Input: part model. Units: mm. Frame: model coordinates. Face numbers are marked on the shaded views. Round coordinates to 2 decimals unless told otherwise and drop trailing zeros. Loops run counter-clockwise (first coordinate to the right, second up) from the corner with the lowest first, then second, coordinate; pieces in that order, holes last. Notation, with made-up numbers: (36.5, 73.25) - (54.5, 73.25) arc R10 cw to (54.5, 89.25) - close; hole circle Ø2 at (69, 3.5). An arc over 180 degrees is marked (long way). One line per question, with ' | ' between items. Start each with the question number.
Item 1: Material intervals for line 1 along Z through (x, y) = (-4.5, 7); line 2 along Y through (x, z) = (-7, -12); line 3 along X through (y, z) = (0, -1), sorted ascending.
Item 2: Section C-C, the plane x = 3. Return loops of the section in (y, z).
Item 3: Section D-D, the plane z = -5. Return loops of the section in (x, y), plus the area to 3 significant figures.
Item 4: Section A-A, the plane y = 11. Return loops of the section in (x, z), plus the area to 3 significant figures.
Item 5: Draft query along X for the marked faces 1, 2, 3 and 4. Return one class per face: pulls with the +X half, pulls with the -X half, needs draft (parallel to the pull), parting line crosses it, or undercut.
Item 6: First-contact query: pin 1 (0.7 mm diameter, centred on x = -9, z = 5.5, fed in from +Y); pin 2 (1.5 mm diameter, centred on y = -0.5, z = 0, fed in from +X); pin 3 (1 mm diameter, centred on x = 9, z = -0.5, fed in from -Y). Flat tips, straight axial feed; report the tip coordinate or a pass-through.
Item 7: Section B-B, the plane y = -3. Return loops of the section in (x, z), plus the area to 3 significant figures.
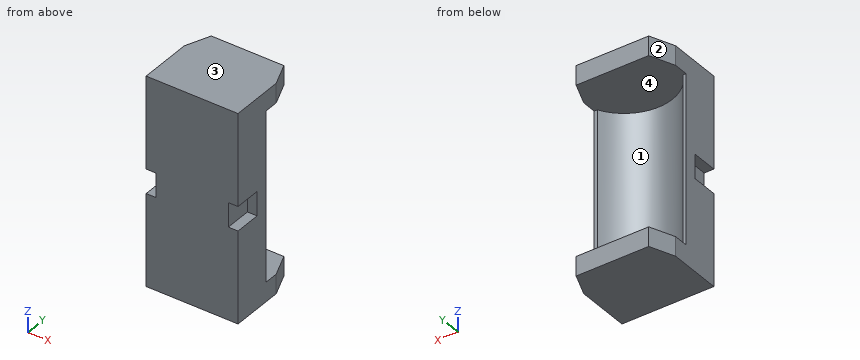
Solid Edge part; units mm, degrees
sketch "Sketch1" plane through (0, 0, 0) normal (0, 0, 1) x (1, 0, 0)
  line L0 (-9.5, -4) -> (-9.5, 4)
  line L1 (-9.5, 4) -> (-8.8569, 4)
  line L2 (8.8569, 4) -> (9.5, 4)
  line L3 (9.5, 4) -> (9.5, -4)
  line L4 (9.5, -4) -> (-9.5, -4)
  arc A0 (8.8569, 4) -> (-8.8569, 4) centre (0, 8.6428) cw
extrude "Protrusion1" add sketch "Sketch1" along normal mid plane 43
sketch "Sketch2" plane through (0, 0, 0) normal (0, -1, 0) x (1, 0, 0)
  line L0 (9.5, 17.5) -> (-9.5, 17.5)
  line L1 (-9.5, 17.5) -> (-9.5, 21.5)
  line L2 (-9.5, 21.5) -> (9.5, 21.5)
  line L3 (9.5, 21.5) -> (9.5, 17.5)
extrude "ExtrudedProtrusion_2" add sketch "Sketch2" against normal blind 12 and the other way blind 2.4828
mirror "Mirror1" about plane through (0, 0, 0) normal (0, 0, 1) of "ExtrudedProtrusion_2"
sketch "Sketch3" plane through (0, 0, 0) normal (0, 0, 1) x (1, 0, 0)
  line L0 (9.5, 7) -> (9.5, 12)
  line L1 (9.5, 12) -> (7.5, 12)
  line L2 (7.5, 12) -> (9.5, 7)
  line L3 (-7.5, 12) -> (-9.5, 7)
  line L4 (-9.5, 7) -> (-9.5, 12)
  line L5 (-9.5, 12) -> (-7.5, 12)
extrude "Cutout1" cut sketch "Sketch3" along normal through all and the other way through all
sketch "Sketch4" plane through (9.5, 1.5, 0) normal (1, 0, 0) x (0, 0, -1)
  line L0 (2.5, -5.5) -> (2.5, 0)
  line L1 (2.5, 0) -> (-2.5, 0)
  line L2 (-2.5, 0) -> (-2.5, -5.5)
  line L3 (-2.5, -5.5) -> (2.5, -5.5)
extrude "ExtrudedCutout_2" cut sketch "Sketch4" against normal blind 2
mirror "Mirror2" about plane through (0, 0, 0) normal (1, 0, 0) of "ExtrudedCutout_2"
Return value:
1) line 1: -21.5 to -17.5, 17.5 to 21.5 | line 2: -4 to 1.5 | line 3: -7.5 to -5.03, 5.03 to 7.5
2) outline: (-4, -21.5) - (12, -21.5) - (12, -17.5) - (-0.9, -17.5) - (-0.9, 17.5) - (12, 17.5) - (12, 21.5) - (-4, 21.5) - close
3) outline: (-9.5, -4) - (9.5, -4) - (9.5, 4) - (8.86, 4) arc R10 cw to (-8.86, 4) - (-9.5, 4) - close | area: 84.3 mm2
4) outline: (-7.9, -21.5) - (7.9, -21.5) - (7.9, -17.5) - (-7.9, -17.5) - close; (-7.9, 17.5) - (7.9, 17.5) - (7.9, 21.5) - (-7.9, 21.5) - close | area: 126 mm2
5) face 1: undercut | face 2: pulls with the -X half | face 3: needs draft | face 4: undercut
6) pin 1: y = 4 | pin 2: x = 7.5 | pin 3: y = 1.5
7) outline: (-9.5, -21.5) - (9.5, -21.5) - (9.5, -2.5) - (7.5, -2.5) - (7.5, 2.5) - (9.5, 2.5) - (9.5, 21.5) - (-9.5, 21.5) - (-9.5, 2.5) - (-7.5, 2.5) - (-7.5, -2.5) - (-9.5, -2.5) - close | area: 797 mm2
